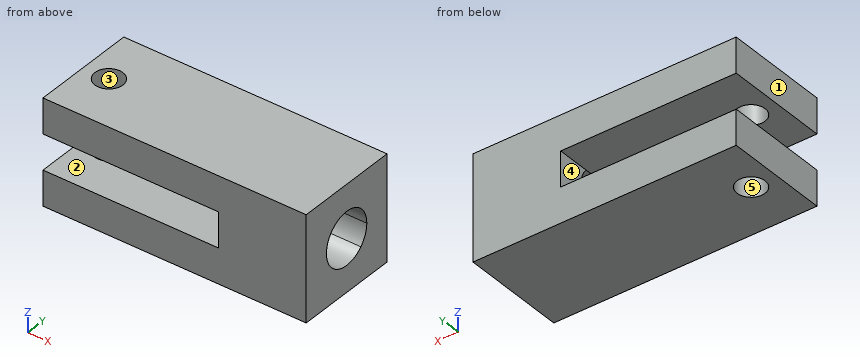
from build123d import *

# Parameters (mm, degrees)
F1_DEPTH = 6
F3_DEPTH = 5
F4_R     = 0.8
F5_DEPTH = 25


with BuildPart() as f1:
    # F0 (on Front) → F1 (new body)
    with BuildSketch(Plane.XZ):
        Polygon((-62.6351881424, 2.6772396487), (-77.6351881424, 2.6772396487), (-77.6351881424, 0.6772396487), (-67.6351881424, 0.6772396487), (-67.6351881424, -1.3227603513), (-77.6351881424, -1.3227603513), (-77.6351881424, -3.3227603513), (-62.6351881424, -3.3227603513), align=None)
    extrude(amount=F1_DEPTH)

    # F2 (on face) → F3 (cut)
    with BuildSketch(Plane.YZ.offset(-62.6351881424)):
        with BuildLine():
            Line((-1.9393398282, -1.3834205231), (-3, -0.3227603513))
            Line((-3, -0.3227603513), (-4.0606601718, -1.3834205231))
            ThreePointArc((-4.0606601718, -1.3834205231), (-3, -1.8227603513), (-1.9393398282, -1.3834205231))
        make_face()
        with BuildLine():
            Line((-1.9393398282, 0.7378998205), (-3, -0.3227603513))
            Line((-3, -0.3227603513), (-1.9393398282, -1.3834205231))
            ThreePointArc((-1.9393398282, -1.3834205231), (-1.6141807012, -0.8967854998), (-1.5, -0.3227603513))
            ThreePointArc((-1.5, -0.3227603513), (-1.6141807012, 0.2512647973), (-1.9393398282, 0.7378998205))
        make_face()
        with BuildLine():
            ThreePointArc((-1.9393398282, 0.7378998205), (-3, 1.1772396487), (-4.0606601718, 0.7378998205))
            Line((-4.0606601718, 0.7378998205), (-3, -0.3227603513))
            Line((-3, -0.3227603513), (-1.9393398282, 0.7378998205))
        make_face()
        with BuildLine():
            Line((-3, -0.3227603513), (-4.0606601718, 0.7378998205))
            ThreePointArc((-4.0606601718, 0.7378998205), (-4.5, -0.3227603513), (-4.0606601718, -1.3834205231))
            Line((-4.0606601718, -1.3834205231), (-3, -0.3227603513))
        make_face()
    extrude(amount=-F3_DEPTH, mode=Mode.SUBTRACT)

    # F4 (on face) → F5 (cut)
    with BuildSketch(Plane(origin=(0, 0, -3.3227603513), x_dir=(1, 0, 0), z_dir=(0, 0, -1))):
        with Locations((-76.1807858944, 3)):
            Circle(F4_R)
    extrude(amount=-F5_DEPTH, mode=Mode.SUBTRACT)


solid = f1.part
The model under review builds one solid part; all positions refer to its coordinate system, in mm. Face numbers are marked on the shaded views. A direction names the side the tool comes from. Coordinates: 2 decimals unless noted, no trailing zeros. Loops run counter-clockwise (first coordinate to the right, second up) from the corner with the lowest first, then second, coordinate; pieces in that order, holes last.
(1) Draft analysis for pull direction X (two halves, no side actions). For the marked faces 1, 2 and 3, state which applies: +X half, -X half, draft (parallel to the pull), parting line (faces both ways), or undercut.
Determined:
face 1: -X half
face 2: draft
face 3: undercut
(2) Consider section A-A, the plane y = -3. Give the boundary of the cut face in (x, z), plus the area to 3 significant figures.
Determined:
outline: (-77.64, -3.32) - (-76.98, -3.32) - (-76.98, -1.32) - (-77.64, -1.32) - close; (-77.64, 0.68) - (-76.98, 0.68) - (-76.98, 2.68) - (-77.64, 2.68) - close; (-75.38, -3.32) - (-62.64, -3.32) - (-62.64, -1.82) - (-67.64, -1.82) - (-67.64, -1.32) - (-75.38, -1.32) - close; (-75.38, 0.68) - (-67.64, 0.68) - (-67.64, 1.18) - (-62.64, 1.18) - (-62.64, 2.68) - (-75.38, 2.68) - close
area: 48.6 mm2
(3) Wall thickness on L1, parallel to X at y = -3, z = 1.8; L2, parallel to Z at x = -73.5, y = -3.9; L3, parallel to Z at x = -63.5, y = -3: over which ranges is each line inside the solid? List them lowest first.
Determined:
L1: x = -77.64 to -76.98, -75.38 to -62.64
L2: z = -3.32 to -1.32, 0.68 to 2.68
L3: z = -3.32 to -1.82, 1.18 to 2.68
(4) Consider section D-D, the plane z = -0.8. Give the boundary of the cut face in (x, y).
Determined:
outline: (-67.64, -6) - (-62.64, -6) - (-62.64, -4.42) - (-67.64, -4.42) - close; (-67.64, -1.58) - (-62.64, -1.58) - (-62.64, 0) - (-67.64, 0) - close
(5) Tool access review of the marked faces 4 and 5: name each direction out of +Z, -Z, +X, -X, +Y, -Y from which nothing blocks a thin tool from reaching the whole face with its end or side.
Determined:
face 4: -X, +Y, -Y
face 5: +Z, -Z
(6) Insertion check: P1, Ø1.3, axis at x = -76.18, y = -3, coming from the +Z side; P2, Ø0.9, axis at y = -0.5, z = -0.5, coming from the -X side. Each pin has a flat end and moves straight along its axis. Give the tip position at first contact, or say it passes through.
Determined:
P1: passes through
P2: stops at x = -67.64
(7) Consider section C-C, the plane z = 1.65. Give the boundary of the cut face in (x, y), plus the area to 3 significant figures.
Determined:
outline: (-77.64, -6) - (-62.64, -6) - (-62.64, 0) - (-77.64, 0) - close; hole circle Ø1.6 at (-76.18, -3)
area: 88.0 mm2
(8) Consider section B-B, the plane x = -71. Give the boundary of the cut face in (y, z), plus the area to 3 significant figures.
Determined:
outline: (-6, -3.32) - (0, -3.32) - (0, -1.32) - (-6, -1.32) - close; (-6, 0.68) - (0, 0.68) - (0, 2.68) - (-6, 2.68) - close
area: 24.0 mm2
